from build123d import *

# Parameters (mm, degrees)
F0_W      = 50.8
F0_H      = 50.8
F1_DEPTH  = 7.62
F2_T      = -1.27
F3_W      = 1.27
F3_H      = 43.18
F4_DEPTH  = 6.35
F5_R      = 1.27
F6_DEPTH  = 25.4
F8_DEPTH  = 6.35
F9_W      = 36.83
F9_H      = 1.27
F10_DEPTH = 6.35
F11_W     = 1.27
F11_H     = 26.6634474313
F12_DEPTH = 6.35
F13_W     = 30.48
F13_H     = 1.27
F14_DEPTH = 6.35
F15_W     = 1.27
F15_H     = 20.3134474313
F16_DEPTH = 6.35
F17_W     = 24.13
F17_H     = 1.27
F18_DEPTH = 6.35
F19_W     = 24.13
F19_H     = 1.27
F20_DEPTH = 6.35
F21_W     = 1.27
F21_H     = 7.6134474313
F22_DEPTH = 6.35
F23_W     = 1.27
F23_H     = 7.6134474313
F24_DEPTH = 6.35
F25_W     = 1.27
F25_H     = 7.6134474313
F26_DEPTH = 6.35
F27_W     = 3.81
F27_H     = 1.27
F28_DEPTH = 6.35
F29_R     = 1.27
F30_DEPTH = 25.4
F31_R     = 1.27
F32_DEPTH = 25.4
F33_R     = 1.27
F34_DEPTH = 25.4


with BuildPart() as f1:
    # F0 (on Top) → F1 (new body)
    with BuildSketch(Plane.XY):
        with Locations((25.4, 25.4)):
            Rectangle(F0_W, F0_H)
    extrude(amount=F1_DEPTH)

    # F2
    f2_openings = [f1.faces().sort_by_distance(p)[0] for p in [
        (25.4, 25.4, 7.62),
    ]]
    offset(amount=F2_T, openings=f2_openings)

    # F3 (on face) → F4 (join)
    with BuildSketch(Plane.XY.offset(1.27)):
        with Locations((6.985, 22.86)):
            Rectangle(F3_W, F3_H)
    extrude(amount=F4_DEPTH)

    # F5 (on face) → F6 (cut)
    with BuildSketch(Plane.XY.offset(1.27)):
        with Locations((3.81, 3.81)):
            Circle(F5_R)
    extrude(amount=-F6_DEPTH, mode=Mode.SUBTRACT)

    # F7 (on face) → F8 (join)
    with BuildSketch(Plane.XY.offset(1.27)):
        Polygon((13.97, 44.45), (7.62, 44.45), (7.62, 43.18), (12.7, 43.18), (12.7, 39.3634474313), (44.45, 39.3634474313), (44.45, 40.6334474313), (13.97, 40.6334474313), align=None)
    extrude(amount=F8_DEPTH)

    # F9 (on face) → F10 (join)
    with BuildSketch(Plane.XY.offset(1.27)):
        with Locations((31.115, 33.6484474313)):
            Rectangle(F9_W, F9_H)
    extrude(amount=F10_DEPTH)

    # F11 (on face) → F12 (join)
    with BuildSketch(Plane.XY.offset(1.27)):
        with Locations((13.335, 19.6817237157)):
            Rectangle(F11_W, F11_H)
    extrude(amount=F12_DEPTH)

    # F13 (on face) → F14 (join)
    with BuildSketch(Plane.XY.offset(1.27)):
        with Locations((29.21, 6.985)):
            Rectangle(F13_W, F13_H)
    extrude(amount=F14_DEPTH)

    # F15 (on face) → F16 (join)
    with BuildSketch(Plane.XY.offset(1.27)):
        with Locations((43.815, 17.7767237157)):
            Rectangle(F15_W, F15_H)
    extrude(amount=F16_DEPTH)

    # F17 (on face) → F18 (join)
    with BuildSketch(Plane.XY.offset(1.27)):
        with Locations((31.115, 27.2984474313)):
            Rectangle(F17_W, F17_H)
    extrude(amount=F18_DEPTH)

    # F19 (on face) → F20 (join)
    with BuildSketch(Plane.XY.offset(1.27)):
        with Locations((26.035, 20.9484474313)):
            Rectangle(F19_W, F19_H)
    extrude(amount=F20_DEPTH)

    # F21 (on face) → F22 (join)
    with BuildSketch(Plane.XY.offset(1.27)):
        with Locations((37.465, 16.5067237157)):
            Rectangle(F21_W, F21_H)
    extrude(amount=F22_DEPTH)

    # F23 (on face) → F24 (join)
    with BuildSketch(Plane.XY.offset(1.27)):
        with Locations((31.115, 11.4267237157)):
            Rectangle(F23_W, F23_H)
    extrude(amount=F24_DEPTH)

    # F25 (on face) → F26 (join)
    with BuildSketch(Plane.XY.offset(1.27)):
        with Locations((24.765, 16.5067237157)):
            Rectangle(F25_W, F25_H)
    extrude(amount=F26_DEPTH)

    # F27 (on face) → F28 (join)
    with BuildSketch(Plane.XY.offset(1.27)):
        Polygon((17.78, 7.62), (19.05, 7.62), (19.05, 15.2334474313), (17.78, 15.2334474313), (17.78, 13.9634474313), align=None)
        with Locations((15.875, 14.5984474313)):
            Rectangle(F27_W, F27_H)
    extrude(amount=F28_DEPTH)

    # F29 (on face) → F30 (cut)
    with BuildSketch(Plane.XY.offset(1.27)):
        with Locations((16.51, 17.7734474313)):
            Circle(F29_R)
    extrude(amount=-F30_DEPTH, mode=Mode.SUBTRACT)

    # F31 (on face) → F32 (cut)
    with BuildSketch(Plane.XY.offset(1.27)):
        with Locations((3.81, 12.7)):
            Circle(F31_R)
    extrude(amount=-F32_DEPTH, mode=Mode.SUBTRACT)

    # F33 (on face) → F34 (cut)
    with BuildSketch(Plane.XY.offset(1.27)):
        with Locations((16.7510975152, 43.2170815766)):
            Circle(F33_R)
    extrude(amount=-F34_DEPTH, mode=Mode.SUBTRACT)


solid = f1.part
Can you work these out from the model? Positions are in its coordinate system, mm. A direction names the side the tool comes from. Give positions to 0.01 mm unless a question says otherwise; leave off trailing zeros. Loops run counter-clockwise (first coordinate to the right, second up) from the corner with the lowest first, then second, coordinate; pieces in that order, holes last. Notation, with made-up numbers: (22.25, -33) -> (63.25, -33) arc R13 cw to (63.25, -29) -> close; hole circle Ø1 at (78, 69). An arc over 180 degrees is marked (long way). Return JSON: item names as keys, results as strings.
Q1. I want a section at B-B, the plane y = 48.5. List the corners of the cut face in (x, z) for me, then the cut area to 3 significant figures.
Checks:
{"outline": "(0, 0) -> (50.8, 0) -> (50.8, 7.62) -> (49.53, 7.62) -> (49.53, 1.27) -> (1.27, 1.27) -> (1.27, 7.62) -> (0, 7.62) -> close", "area": "80.6 mm2"}
Q2. I want a section at C-C, the plane x = 35. List the corners of the cut face in (y, z) for me.
Checks:
{"outline": "(0, 0) -> (50.8, 0) -> (50.8, 7.62) -> (49.53, 7.62) -> (49.53, 1.27) -> (40.63, 1.27) -> (40.63, 7.62) -> (39.36, 7.62) -> (39.36, 1.27) -> (34.28, 1.27) -> (34.28, 7.62) -> (33.01, 7.62) -> (33.01, 1.27) -> (27.93, 1.27) -> (27.93, 7.62) -> (26.66, 7.62) -> (26.66, 1.27) -> (21.58, 1.27) -> (21.58, 7.62) -> (20.31, 7.62) -> (20.31, 1.27) -> (7.62, 1.27) -> (7.62, 7.62) -> (6.35, 7.62) -> (6.35, 1.27) -> (1.27, 1.27) -> (1.27, 7.62) -> (0, 7.62) -> close"}
Q3. For pin 1 Ø1.1 at (x, y) = (15.5, 9.5) entering from +Z, with a flat end and sliding along its axis, tell me the tip position at first contact or that it passes through.
Checks:
{"pin 1": "stops at z = 1.27"}
Q4. On a 3-axis mill with a long thin cutter (end or side, diameter ignored), from which of +Z, -Z, +X, -X, +Y, -Y can I reach the whole of each face in a straight line? I mean faces 4 (the face through (15.57, 18.63, 0.64)), 5 (the face through (31, 20.313, 4)). Say none if no direction works.
Checks:
{"face 4": "+Z, -Z", "face 5": "+Z"}
Q5. We'd pull the mould along X, two halves only. Please class faces 1 (the face through (10, 43.18, 4)), 2 (the face through (25, 26, 0)), 3 (the face through (31, 15.233, 4)): released by +X, released by -X, zero draft, split by the parting line, or undercut.
Checks:
{"face 1": "undercut", "face 2": "zero draft", "face 3": "undercut"}
Q6. I need wall thicknesses on probe 1 along X at (y, z) = (23, 6); probe 2 along X at (y, z) = (31, 5); probe 3 along X at (y, z) = (21.5, 3.75). Which ranges of each line are inside material? Lowest first, please.
Checks:
{"probe 1": "x = 0 to 1.27, 6.35 to 7.62, 12.7 to 13.97, 43.18 to 44.45, 49.53 to 50.8", "probe 2": "x = 0 to 1.27, 6.35 to 7.62, 12.7 to 13.97, 49.53 to 50.8", "probe 3": "x = 0 to 1.27, 6.35 to 7.62, 12.7 to 38.1, 43.18 to 44.45, 49.53 to 50.8"}
Q7. I want a section at D-D, the plane z = 3.25. Count the separate pieces of the cut face and the enclosed holes in it, then the cut area to 3 significant figures.
Checks:
{"separate pieces": "1", "enclosed holes": "2", "area": "608 mm2"}
Q8. I want a section at A-A, the plane y = 3.81. List the corners of the cut face in (x, z) for me, then the cut area to 3 significant figures.
Checks:
{"outline": "(0, 0) -> (2.54, 0) -> (2.54, 1.27) -> (1.27, 1.27) -> (1.27, 7.62) -> (0, 7.62) -> close; (5.08, 0) -> (50.8, 0) -> (50.8, 7.62) -> (49.53, 7.62) -> (49.53, 1.27) -> (7.62, 1.27) -> (7.62, 7.62) -> (6.35, 7.62) -> (6.35, 1.27) -> (5.08, 1.27) -> close", "area": "85.5 mm2"}
